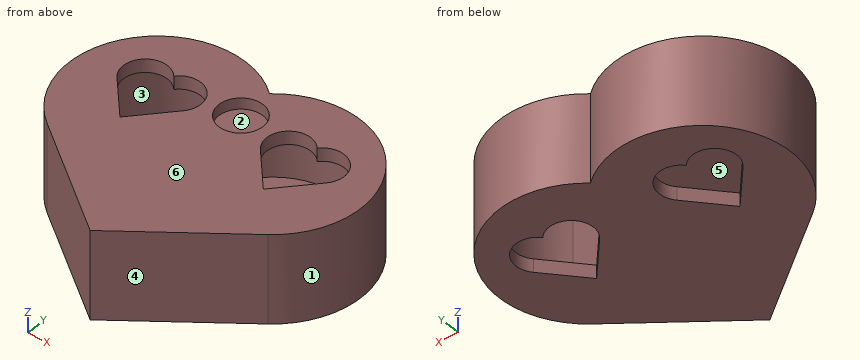
```python
from build123d import *

# Parameters (mm, degrees)
EXTRUDE_1_DEPTH     = 10
SKETCH_2_R          = 5
CUT_EXTRUDE_1_DEPTH = 2.5
CUT_EXTRUDE_2_DEPTH = 7
CUT_EXTRUDE_3_DEPTH = 20


with BuildPart() as part:
    # 草圖1 → 填料-伸長1 (new, symmetric)
    with BuildSketch(Plane.XY):
        with BuildLine():
            Line((-24.197007139, 36.923558221), (0.802992861, 18.124320865))
            Line((0.802992861, 18.124320865), (25.802992861, 36.923558221))
            ThreePointArc((25.802992861, 36.923558221), (29.390613552, 65.414346162), (0.802992861, 68.124320865))
            ThreePointArc((0.802992861, 68.124320865), (-27.78462783, 65.414346162), (-24.197007139, 36.923558221))
        make_face()
    extrude(amount=EXTRUDE_1_DEPTH, both=True)

    # 草圖2 → 除料-伸長1 (cut)
    with BuildSketch(Plane.XY.offset(10)):
        with Locations((0.802992861, 60.124320865)):
            Circle(SKETCH_2_R)
    extrude(amount=-CUT_EXTRUDE_1_DEPTH, mode=Mode.SUBTRACT)

    # 草圖3 → 除料-伸長2 (cut, symmetric)
    with BuildSketch(Plane.XY):
        with BuildLine():
            Line((0.802992861, 20.124320865), (23.302992861, 45.282290118))
            ThreePointArc((23.302992861, 45.282290118), (22.043474428, 66.532077134), (0.802992861, 65.124320865))
            ThreePointArc((0.802992861, 65.124320865), (-20.437488706, 66.532077134), (-21.697007139, 45.282290118))
            Line((-21.697007139, 45.282290118), (0.802992861, 20.124320865))
        make_face()
    extrude(amount=CUT_EXTRUDE_2_DEPTH, both=True, mode=Mode.SUBTRACT)

    # 草圖4 → 除料-伸長3 (cut)
    with BuildSketch(Plane(origin=(0, 0, -10), x_dir=(-1, 0, 0), z_dir=(0, 0, -1))):
        with BuildLine():
            Line((7.923932244, 54.791149812), (15.423932244, 46.405160061))
            Line((15.423932244, 46.405160061), (22.923932244, 54.791149812))
            ThreePointArc((22.923932244, 54.791149812), (22.504092766, 61.874412151), (15.423932244, 61.405160061))
            ThreePointArc((15.423932244, 61.405160061), (8.343771721, 61.874412151), (7.923932244, 54.791149812))
        make_face()
        with BuildLine():
            Line((-17.029917966, 46.405160061), (-24.529917966, 54.791149812))
            ThreePointArc((-24.529917966, 54.791149812), (-24.110078488, 61.874412151), (-17.029917966, 61.405160061))
            ThreePointArc((-17.029917966, 61.405160061), (-9.949757443, 61.874412151), (-9.529917966, 54.791149812))
            Line((-9.529917966, 54.791149812), (-17.029917966, 46.405160061))
        make_face()
    extrude(amount=-CUT_EXTRUDE_3_DEPTH, mode=Mode.SUBTRACT)


solid = part.part
```
Verification items for the finished model (mm, model axes). Face numbers are marked on the shaded views. A direction names the side the tool comes from. Give positions to 0.01 mm unless a question says otherwise; leave off trailing zeros. Loops run counter-clockwise (first coordinate to the right, second up) from the corner with the lowest first, then second, coordinate; pieces in that order, holes last. Notation, with made-up numbers: M 51,25.25 L 100,25.25 A22 cw 100,57.25 Z; hole C 33.5,11.25 d7. An arc over 180 degrees is marked long. Return JSON: item names as keys, results as strings.
1) Section check A-A, the plane x = -9. Enter the section's corners in (y, z).
Findings:
{"outline": "M 25.5,-10 L 53.59,-10 L 53.59,-7 L 31.09,-7 L 31.09,7 L 53.59,7 L 53.59,10 L 25.5,10 Z; M 62.36,-10 L 72.65,-10 L 72.65,10 L 62.36,10 L 62.36,7 L 70.2,7 L 70.2,-7 L 62.36,-7 Z"}
2) Section check B-B, the plane y = 57. Enter the section's corners in (x, z), and give its area (3 significant figures).
Findings:
{"outline": "M -31.75,-10 L -24.07,-10 L -24.07,-7 L -25.42,-7 L -25.42,7 L -24.07,7 L -24.07,10 L -31.75,10 Z; M -6.78,-10 L 8.38,-10 L 8.38,-7 L -6.78,-7 Z; M -6.78,7 L 8.38,7 L 8.38,10 L 4.71,10 L 4.71,7.5 L -3.1,7.5 L -3.1,10 L -6.78,10 Z; M 25.67,-10 L 33.36,-10 L 33.36,10 L 25.67,10 L 25.67,7 L 27.02,7 L 27.02,-7 L 25.67,-7 Z", "area": "341 mm2"}
3) Material ranges on L1, parallel to Z at x = -2.5, y = 43; L2, parallel to X at y = 62, z = -8.5; L3, parallel to X at y = 51, z = 7.25, recorded low to high. Write a range as [from, to].
Findings:
{"L1": "z = [-10, -7], [7, 10]", "L2": "x = [-29.99, -22.36], [-16.04, -14.81], [-8.49, 10.1], [16.42, 17.64], [23.96, 31.6]", "L3": "x = [-32.09, -19.53], [-11.31, 12.92], [21.14, 33.69]"}
4) Gauge pin test, flat ends, axial feed: P1, Ø1.5, axis at x = -16.5, z = -4, coming from the +Y side; P2, Ø9, axis at x = 0.8, y = 60.12, coming from the +Z side; P3, Ø6, axis at y = 66, z = 2.5, coming from the +X side. Record the tip position at first contact, or that the pin passes through.
Findings:
{"P1": "stops at y = 72.59", "P2": "stops at z = 7.5", "P3": "stops at x = 31.05"}
5) Tool access check on the marked faces 1, 2 and 3. Record the directions out of +Z, -Z, +X, -X, +Y, -Y that give a thin tool (end or side, any length) a straight path to the whole face; none if there is none.
Findings:
{"face 1": "+Z, -Z", "face 2": "+Z", "face 3": "none"}
6) Section check C-C, the plane z = 8.5. Enter the section's corners in (x, y).
Findings:
{"outline": "M -24.2,36.92 L 0.8,18.12 L 25.8,36.92 A20 ccw long 0.8,68.12 A20 ccw long Z; hole M -22.92,54.79 L -15.42,46.41 L -7.92,54.79 A5 ccw long -15.42,61.41 A5 ccw long Z; hole C 0.8,60.12 d10; hole M 9.53,54.79 L 17.03,46.41 L 24.53,54.79 A5 ccw long 17.03,61.41 A5 ccw long Z"}
7) Section check D-D, the plane y = 23. Enter the section's corners in (x, z), and give its area (3 significant figures).
Findings:
{"outline": "M -5.68,-10 L 7.29,-10 L 7.29,10 L -5.68,10 Z; hole M -1.77,-7 L 3.37,-7 L 3.37,7 L -1.77,7 Z", "area": "187 mm2"}
8) Mould release check, pull along Y, two halves, no side actions. Record for the marked faces 4, 5 and 6: released by +Y, released by -Y, zero draft, split by the parting line, or undercut.
Findings:
{"face 4": "released by -Y", "face 5": "undercut", "face 6": "zero draft"}
